Geometry: final body of the model. Coordinates: model frame, mm. Round coordinates to 2 decimals unless told otherwise and drop trailing zeros. Loops run counter-clockwise (first coordinate to the right, second up) from the corner with the lowest first, then second, coordinate; pieces in that order, holes last. Notation, with made-up numbers: (13.5, 70.25) - (67.5, 70.25) arc R19 ccw to (67.5, 98.25) - close; hole circle Ø7 at (-34, 56). An arc over 180 degrees is marked (long way). Answer in a Markdown table with one row per item. Add a question column.
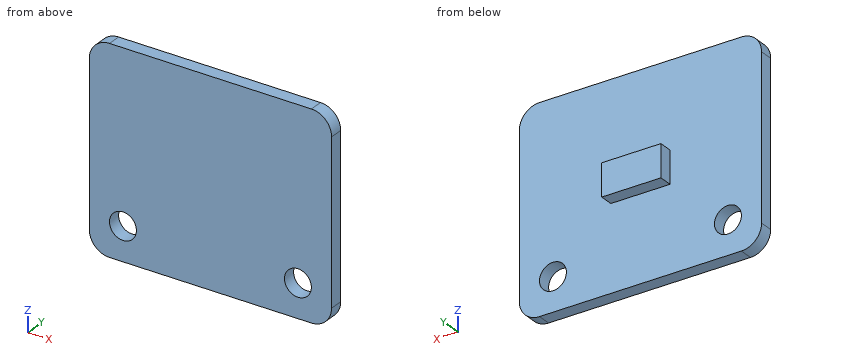
from build123d import *

# Parameters (mm, degrees)
SKETCH1_W           = 18
SKETCH1_H           = 15
SKETCH1_R           = 1
BOSS_EXTRUDE1_DEPTH = 1
SKETCH1_4_W         = 4.4
SKETCH1_4_H         = 2.4
BOSS_EXTRUDE2_DEPTH = 1
FILLET1_R           = 1.5


with BuildPart() as part:
    # Sketch1 → Boss-Extrude1 (new body)
    with BuildSketch(Plane(origin=(0, 0, 0), x_dir=(1, 0, 0), z_dir=(0, 1, 0))):
        Rectangle(SKETCH1_W, SKETCH1_H)
        with Locations(Location((-6.5, 5, 0), (0, 0, 270))):
            Circle(SKETCH1_R, mode=Mode.SUBTRACT)
        with Locations(Location((6.5, 5, 0), (0, 0, 270))):
            Circle(SKETCH1_R, mode=Mode.SUBTRACT)
    extrude(amount=-BOSS_EXTRUDE1_DEPTH)

    # Sketch1_4 → Boss-Extrude2 (add)
    with BuildSketch(Plane(origin=(0, 0, 0), x_dir=(1, 0, 0), z_dir=(0, 1, 0))):
        Rectangle(SKETCH1_4_W, SKETCH1_4_H)
    extrude(amount=BOSS_EXTRUDE2_DEPTH)

    # Fillet1
    fillet1_edges = [part.edges().sort_by_distance(p)[0] for p in [
        (-9, -0.5, 7.5),
        (9, -0.5, 7.5),
        (9, -0.5, -7.5),
        (-9, -0.5, -7.5),
    ]]
    fillet(fillet1_edges, radius=FILLET1_R)


solid = part.part
1) Section C-C, the plane z = -5. Return the cut outline in (x, y), and give its area (3 significant figures).
2) Section D-D, the plane x = -1.75. Return the cut outline in (y, z).
3) Contact query for a flat-ended pin moving along its axis: pin 1 Ø0.5 at (x, y) = (0, 0.5) entering from -Z. Output: stop coordinate, or through.
4) Section A-A, the plane y = -0.45. Return the cut outline in (x, z).
5) Section B-B, the plane x = 6.5. Return the cut outline in (y, z), and give its area (3 significant figures).
6) Material intervals for line 1 along X through (y, z) = (-0.45, -5); line 2 along X through (y, z) = (0.85, -1); line 3 along Y through (x, z) = (0, 2.25), sorted ascending. Write a range as from..to.
Evaluation:
| question | item | result |
|---|---|---|
| 1 | outline | (-9, -1) - (-7.5, -1) - (-7.5, 0) - (-9, 0) - close; (-5.5, -1) - (5.5, -1) - (5.5, 0) - (-5.5, 0) - close; (7.5, -1) - (9, -1) - (9, 0) - (7.5, 0) - close |
| 1 | area | 14.0 mm² |
| 2 | outline | (-1, -7.5) - (0, -7.5) - (0, -1.2) - (1, -1.2) - (1, 1.2) - (0, 1.2) - (0, 7.5) - (-1, 7.5) - close |
| 3 | pin 1 | stops at z = -1.2 |
| 4 | outline | (-9, -6) arc R1.5 ccw to (-7.5, -7.5) - (7.5, -7.5) arc R1.5 ccw to (9, -6) - (9, 6) arc R1.5 ccw to (7.5, 7.5) - (-7.5, 7.5) arc R1.5 ccw to (-9, 6) - close; hole circle Ø2 at (-6.5, -5); hole circle Ø2 at (6.5, -5) |
| 5 | outline | (-1, -7.5) - (0, -7.5) - (0, -6) - (-1, -6) - close; (-1, -4) - (0, -4) - (0, 7.5) - (-1, 7.5) - close |
| 5 | area | 13.0 mm² |
| 6 | line 1 | x = -9..-7.5, -5.5..5.5, 7.5..9 |
| 6 | line 2 | x = -2.2..2.2 |
| 6 | line 3 | y = -1..0 |
